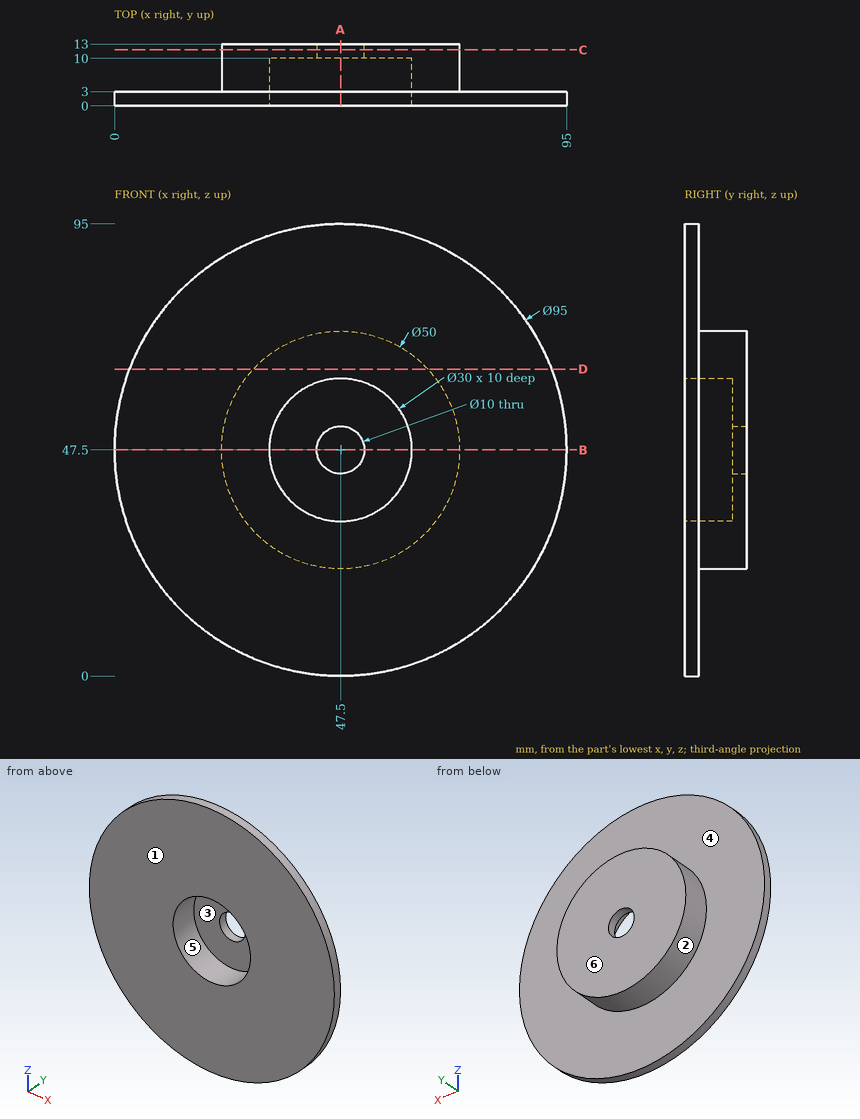
Verification items for this drawing (mm, ordinates from the low corner). A direction names the side the tool comes from. Coordinates: 2 decimals unless noted, no trailing zeros. Write each loop counter-clockwise with the first axis right and the second up, starting at its lowest first coordinate (ties: lowest second). Pieces come first, ordered by that corner, then holes. Notation, with made-up numbers: M -37.75,2 L -5.75,2 A34 cw -5.75,32 Z; hole C 45,50.25 d5. An arc over 180 degrees is marked long. Answer as a JSON object with one key per item and string values. Group by question number.
(1) Cross-section at C-C, the plane y = 11.75. Record the cut outline in (x, z).
(2) Release check for a two-part mould opening along Z. For the marked faces 1, 2 and 3 record: +Z half, -Z half, draft (parallel to the pull), parting line (faces both ways), or undercut.
(3) Material ranges on line 1 (Z direction, x = 47.5, y = 8); line 2 (Y direction, x = 79.5, z = 32); line 3 (Z direction, x = 47.5, y = 10.7), recorded low to high.
(4) Gauge pin test, flat ends, axial feed: pin 1 (9 mm diameter, centred on x = 46.5, z = 54, fed in from -Y); pin 2 (1 mm diameter, centred on x = 19, z = 17, fed in from +Y); pin 3 (1.5 mm diameter, centred on y = 2, z = 55.5, fed in from +X). Record the tip position at first contact, or that the pin passes through.
(5) Cross-section at A-A, the plane x = 47.5. Record the cut outline in (y, z).
(6) Cross-section at B-B, the plane z = 47.5. Record the cut outline in (x, y).
(7) Cross-section at D-D, the plane z = 64.5. Record the cut outline in (x, y).
(8) Tool access check on the marked faces 4, 5 and 6. Record the directions out of +Z, -Z, +X, -X, +Y, -Y that give a thin tool (end or side, any length) a straight path to the whole face; none if there is none.
Reply:
{
 "1": {"outline": "C 47.5,47.5 d50; hole C 47.5,47.5 d10"},
 "2": {"face 1": "draft", "face 2": "parting line", "face 3": "undercut"},
 "3": {"line 1": "22.5 to 32.5, 62.5 to 72.5", "line 2": "0 to 3", "line 3": "22.5 to 42.5, 52.5 to 72.5"},
 "4": {"pin 1": "y = 10", "pin 2": "y = 3", "pin 3": "x = 94.44"},
 "5": {"outline": "M 0,0 L 3,0 L 3,22.5 L 13,22.5 L 13,42.5 L 10,42.5 L 10,32.5 L 0,32.5 Z; M 0,62.5 L 10,62.5 L 10,52.5 L 13,52.5 L 13,72.5 L 3,72.5 L 3,95 L 0,95 Z"},
 "6": {"outline": "M 0,0 L 32.5,0 L 32.5,10 L 42.5,10 L 42.5,13 L 22.5,13 L 22.5,3 L 0,3 Z; M 52.5,10 L 62.5,10 L 62.5,0 L 95,0 L 95,3 L 72.5,3 L 72.5,13 L 52.5,13 Z"},
 "7": {"outline": "M 3.15,0 L 91.85,0 L 91.85,3 L 65.83,3 L 65.83,13 L 29.17,13 L 29.17,3 L 3.15,3 Z"},
 "8": {"face 4": "+Y", "face 5": "-Y", "face 6": "+Z, -Z, +X, -X, +Y"}
}
